The model under review builds one solid part; all positions refer to its coordinate system, in mm. Face numbers are marked on the shaded views. Coordinates: 2 decimals unless noted, no trailing zeros. Loops run counter-clockwise (first coordinate to the right, second up) from the corner with the lowest first, then second, coordinate; pieces in that order, holes last. Notation, with made-up numbers: (-18, 47.25) - (23, 47.25) arc R19 ccw to (23, 83.25) - close; hole circle Ø10 at (-33, 63.5). An arc over 180 degrees is marked (long way). Use a Markdown table: item, result. Add a question column.
1) The part is to be moulded in two halves that separate along X. For the marked faces 1, 2 and 3, say which applies: pulls with the +X half, pulls with the -X half, needs draft (parallel to the pull), parting line crosses it, or undercut.
2) Add section C-C, the plane y = 6. Give the boundary of the cut face in (x, z), and give its area (3 significant figures).
3) Add section A-A, the plane z = 12.5. Give the boundary of the cut face in (x, y).
4) To check wall thickness, follow L1, parallel to X at y = 7.5, z = 12.5; L2, parallel to Z at x = 0, y = 2; L3, parallel to Z at x = 6.5, y = 3. State the ranges of each line that lie inside material, in increasing order. Write a range as [from, to].
5) Clearance check with a flat-ended pin moving along its axis: pin 1 (16 mm diameter, centred on x = 0, z = 12.5, fed in from -Y). State where the tip first meets the part, or that it passes through.
6) Add section B-B, the plane x = 0. Give the boundary of the cut face in (y, z).
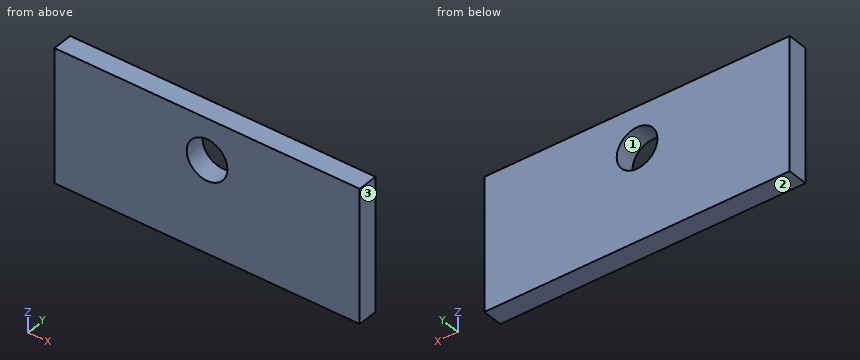
```python
from build123d import *

# Parameters (mm, degrees)
SKETCH1_W               = 150
SKETCH1_H               = 65
BOSS_EXTRUDE1_DEPTH     = 10
SKETCH2_R               = 10
CUT_EXTRUDE2_DEPTH      = 11
CUT_EXTRUDE2_DEPTH_BACK = 1


with BuildPart() as part:
    # Sketch1 → Boss-Extrude1 (new body)
    with BuildSketch(Plane(origin=(0, 0, 0), x_dir=(1, 0, 0), z_dir=(0, 1, 0))):
        Rectangle(SKETCH1_W, SKETCH1_H)
    extrude(amount=BOSS_EXTRUDE1_DEPTH)

    # Sketch2 → Cut-Extrude2 (cut, two sides)
    with BuildSketch(Plane(origin=(0, 0, 0), x_dir=(1, 0, 0), z_dir=(0, 1, 0))) as cut_extrude2_sk:
        with Locations((0, -12.5)):
            Circle(SKETCH2_R)
    extrude(amount=CUT_EXTRUDE2_DEPTH, mode=Mode.SUBTRACT)
    extrude(cut_extrude2_sk.sketch, amount=-CUT_EXTRUDE2_DEPTH_BACK, mode=Mode.SUBTRACT)


solid = part.part
```
From the geometry:
| question | item | result |
|---|---|---|
| 1 | face 1 | undercut |
| 1 | face 2 | needs draft |
| 1 | face 3 | pulls with the +X half |
| 2 | outline | (-75, -32.5) - (75, -32.5) - (75, 32.5) - (-75, 32.5) - close; hole circle Ø20 at (0, 12.5) |
| 2 | area | 9,440 mm^2 |
| 3 | outline | (-75, 0) - (-10, 0) - (-10, 10) - (-75, 10) - close; (10, 0) - (75, 0) - (75, 10) - (10, 10) - close |
| 4 | L1 | x = [-75, -10], [10, 75] |
| 4 | L2 | z = [-32.5, 2.5], [22.5, 32.5] |
| 4 | L3 | z = [-32.5, 4.9], [20.1, 32.5] |
| 5 | pin 1 | passes through |
| 6 | outline | (0, -32.5) - (10, -32.5) - (10, 2.5) - (0, 2.5) - close; (0, 22.5) - (10, 22.5) - (10, 32.5) - (0, 32.5) - close |
